Check sheet for the drawn part. Datum: minimum x, y, z corner. Units: mm. Coordinates: 2 decimals unless noted, no trailing zeros. Order: outer loops, then holes, each group sorted by start corner. A loop starts at its lowest first (then second) coordinate and runs counter-clockwise, first axis right, second up.
1. Thickness scan on line 1 (Z direction, x = 102, y = 2.15); line 2 (X direction, y = 2.3, z = 55) (1 decimal); line 3 (X direction, y = 0.9, z = 87.5). Record the ranges inside material, lowest first.
2. Cross-section at C-C (y = 1.55). Enter the section's corners in (x, z).
3. Gauge pin test, flat end, axial feed: pin 1 Ø1.5 at (x, y) = (17, 1.5) entering from -Z. Record the tip position at first contact, or that the pin passes through.
4. Cross-section at A-A (z = 70). Enter the section's corners in (x, y).
5. Cross-section at B-B (x = 70). Enter the section's corners in (y, z).
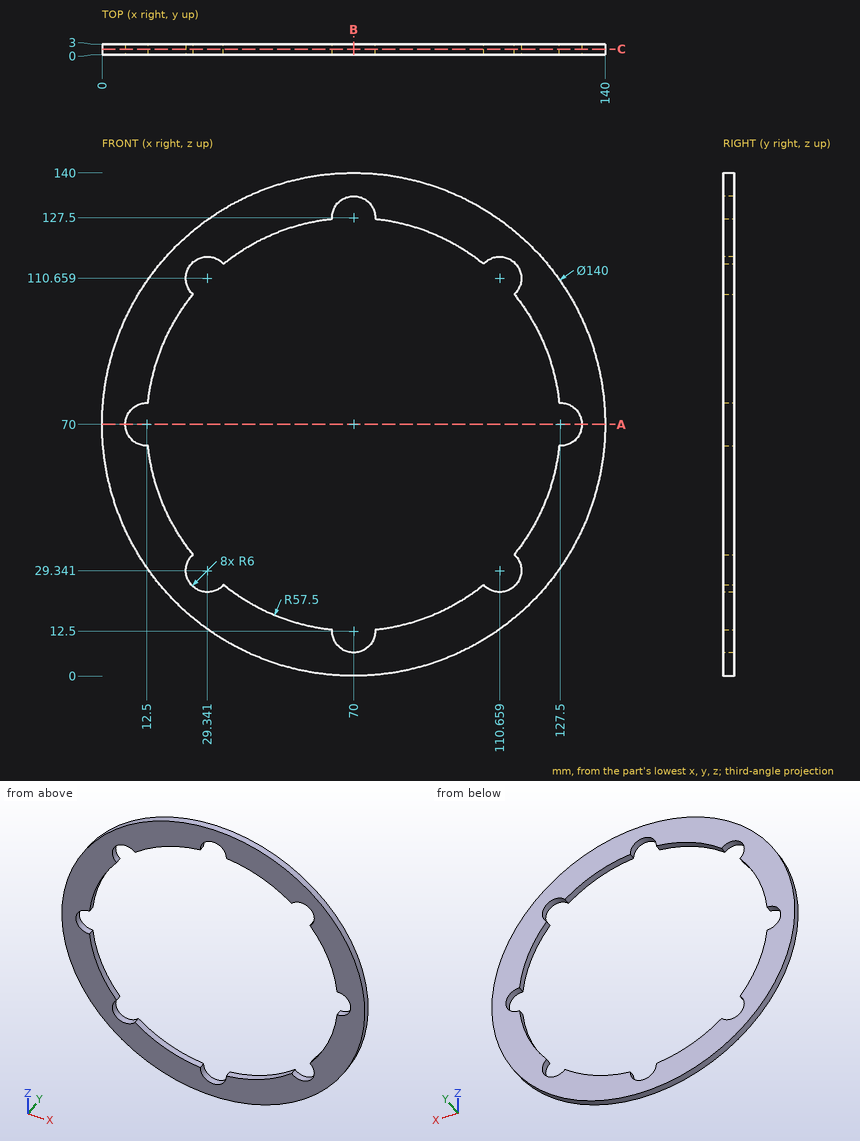
Data:
1. line 1: z = 7.74 to 22.23, 117.77 to 132.26
1. line 2: x = 1.6 to 14.5, 125.5 to 138.4
1. line 3: x = 2.22 to 15.23, 124.77 to 137.78
2. outline: circle Ø140 at (70, 70); hole (12.81, 64.01) arc R57.5 ccw to (25.33, 33.8) arc R6 ccw (long way) to (33.8, 25.33) arc R57.5 ccw to (64.01, 12.81) arc R6 ccw (long way) to (75.99, 12.81) arc R57.5 ccw to (106.2, 25.33) arc R6 ccw (long way) to (114.67, 33.8) arc R57.5 ccw to (127.19, 64.01) arc R6 ccw (long way) to (127.19, 75.99) arc R57.5 ccw to (114.67, 106.2) arc R6 ccw (long way) to (106.2, 114.67) arc R57.5 ccw to (75.99, 127.19) arc R6 ccw (long way) to (64.01, 127.19) arc R57.5 ccw to (33.8, 114.67) arc R6 ccw (long way) to (25.33, 106.2) arc R57.5 ccw to (12.81, 75.99) arc R6 ccw (long way) to start
3. pin 1: stops at z = 23.42
4. outline: (0, 0) - (6.5, 0) - (6.5, 3) - (0, 3) - close; (133.5, 0) - (140, 0) - (140, 3) - (133.5, 3) - close
5. outline: (0, 0) - (3, 0) - (3, 6.5) - (0, 6.5) - close; (0, 133.5) - (3, 133.5) - (3, 140) - (0, 140) - close
